Read the model definition and answer for the solid it produces. Units are mm, in the model's axes. Face numbers are marked on the shaded views. A direction names the side the tool comes from. Coordinates: 2 decimals unless noted, no trailing zeros. Loops run counter-clockwise (first coordinate to the right, second up) from the corner with the lowest first, then second, coordinate; pieces in that order, holes last. Notation, with made-up numbers: M -37,72 L -17,72 A17 cw -17,79 Z; hole C 50.25,3.5 d2. An arc over 180 degrees is marked long. Put each result on its own line as item: value.
from build123d import *

# Parameters (mm, degrees)
BOSS_EXTRUDE1_DEPTH = 80.4
SKETCH2_R           = 3.175
CUT_EXTRUDE1_DEPTH  = 4.175
SKETCH3_R           = 1.5
SKETCH3_R_2         = 3
CUT_EXTRUDE2_DEPTH  = 52.175


with BuildPart() as part:
    # Sketch1 → Boss-Extrude1 (new body)
    with BuildSketch(Plane.XY):
        Polygon((0, 0), (3.175, 0), (3.175, 48), (45.475, 48), (45.475, 51.175), (0, 51.175), align=None)
    extrude(amount=BOSS_EXTRUDE1_DEPTH)

    # Sketch2 → Cut-Extrude1 (cut, through all)
    with BuildSketch(Plane(origin=(3.175, 0, 0), x_dir=(0, 0, -1), z_dir=(1, 0, 0))):
        with Locations((-70.875, 12.7)):
            Circle(SKETCH2_R)
        with Locations((-9.525, 12.7)):
            Circle(SKETCH2_R)
    extrude(amount=-CUT_EXTRUDE1_DEPTH, mode=Mode.SUBTRACT)

    # Sketch3 → Cut-Extrude2 (cut, through all)
    with BuildSketch(Plane(origin=(0, 51.175, 0), x_dir=(1, 0, 0), z_dir=(0, 1, 0))):
        with Locations((39.825, -55.7)):
            Circle(SKETCH3_R)
        with Locations((8.825, -55.7)):
            Circle(SKETCH3_R)
        with Locations((8.825, -24.7)):
            Circle(SKETCH3_R)
        with Locations((39.825, -24.7)):
            Circle(SKETCH3_R)
        with Locations((24.325, -40.2)):
            Circle(SKETCH3_R_2)
    extrude(amount=-CUT_EXTRUDE2_DEPTH, mode=Mode.SUBTRACT)


solid = part.part
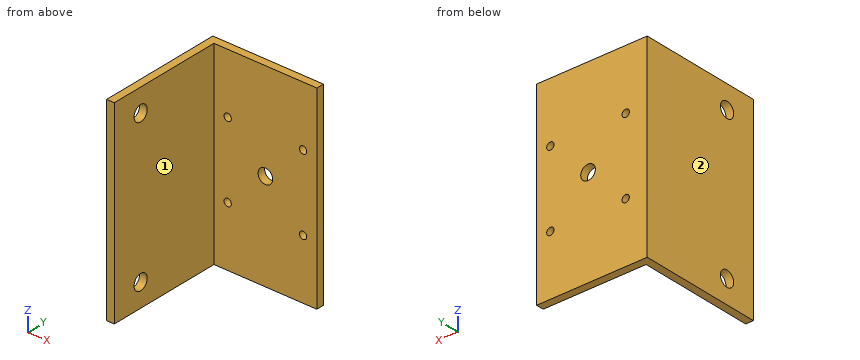
1) Given pin 1 Ø5 at (x, z) = (28.5, 51) entering from -Y; pin 2 Ø8 at (y, z) = (42, 38.5) entering from +X (3 decimals), each flat-ended and moving along its own axis, determine where each tip first touches the part or whether it passes through.
Answer list:
pin 1: stops at y = 48
pin 2: stops at x = 3.175
2) Find section A-A, the plane z = 40.2. Write down the section's boundary in (x, y) (3 decimals).
Answer list:
outline: M 0,0 L 3.175,0 L 3.175,48 L 21.325,48 L 21.325,51.175 L 0,51.175 Z; M 27.325,48 L 45.475,48 L 45.475,51.175 L 27.325,51.175 Z
3) Find section D-D, the plane x = 30. Write down the section's boundary in (y, z) (3 decimals).
Answer list:
outline: M 48,0 L 51.175,0 L 51.175,80.4 L 48,80.4 Z
4) Straight lines are drawn through the part: line 1 (X direction, y = 50, z = 24.7) (3 decimals); line 2 (X direction, y = 40, z = 53) (3 decimals); line 3 (Y direction, x = 8, z = 21) (3 decimals). For each, find the intervals that lie inside material, in ascending order. Write a range as [from, to].
Answer list:
line 1: x = [0, 7.325], [10.325, 38.325], [41.325, 45.475]
line 2: x = [0, 3.175]
line 3: y = [48, 51.175]
5) Which of the six approach directions +Z, -Z, +X, -X, +Y, -Y give full straight-line access (tool end or side, diameter ignored) to the marked faces 1 and 2?
Answer list:
face 1: +Z, -Z, +X, -Y
face 2: +Z, -Z, -X, +Y, -Y
6) Find section B-B, the plane z = 55.7. Write down the section's boundary in (x, y) (3 decimals).
Answer list:
outline: M 0,0 L 3.175,0 L 3.175,48 L 7.325,48 L 7.325,51.175 L 0,51.175 Z; M 10.325,48 L 38.325,48 L 38.325,51.175 L 10.325,51.175 Z; M 41.325,48 L 45.475,48 L 45.475,51.175 L 41.325,51.175 Z
7) Find section C-C, the plane y = 12.7. Write down the section's boundary in (x, z) (3 decimals), plus the area to 3 significant figures.
Answer list:
outline: M 0,0 L 3.175,0 L 3.175,6.35 L 0,6.35 Z; M 0,12.7 L 3.175,12.7 L 3.175,67.7 L 0,67.7 Z; M 0,74.05 L 3.175,74.05 L 3.175,80.4 L 0,80.4 Z
area: 215 mm^2
